For this review, take the finished solid that the model builds, in its own axes (mm). Coordinates: 2 decimals unless noted, no trailing zeros. Write each loop counter-clockwise with the first axis right and the second up, starting at its lowest first coordinate (ties: lowest second). Pieces come first, ordered by that corner, then holes. Notation, with made-up numbers: (-29, 33.5) -> (22, 33.5) arc R29 ccw to (22, 54.5) -> close; hole circle Ø1 at (-37, -15.5). An arc over 180 degrees is marked (long way). One line per item, written item: value. Start each with the question number.
1) Add section B-B (z = -226.5). State the section outline as (x, y) points, and give its area (3 significant figures).
2) For pin 1 Ø1.9 at (x, z) = (1.5, -552.5) entering from +Y; pin 2 Ø1.9 at (x, y) = (3, 617) entering from +Z, all flat-tipped, find the tip position at first contact; note any pin that passes through.
3) Add section A-A (x = 5). State how many separate pieces and enclosed holes the cut face has, and give its area (3 significant figures).
4) For probe 1 along Y at (x, z) = (1.75, -133.35); probe 2 along Y at (x, z) = (0.75, -596.5); probe 3 along Z at (x, y) = (5.75, 587), list the stretches that pass through material, from the lowest coordinate up. Write a range as from..to.
from build123d import *

# Parameters (mm, degrees)
SKETCH1_R           = 2.45745
BOSS_EXTRUDE1_DEPTH = 6.35
SKETCH3_R           = 2.45745
CUT_EXTRUDE2_DEPTH  = 1034.724611538


with BuildPart() as part:
    # Sketch1 → Boss-Extrude1 (new body)
    with BuildSketch(Plane(origin=(0, 0, 0), x_dir=(0, 0, -1), z_dir=(1, 0, 0))):
        with BuildLine():
            Line((457.2, 546.1), (755.65, 546.1))
            ThreePointArc((755.65, 546.1), (760.140128061, 544.240128061), (762, 539.75))
            Line((762, 539.75), (762, 6.35))
            ThreePointArc((762, 6.35), (760.140128061, 1.859871939), (755.65, 0))
            Line((755.65, 0), (6.35, 0))
            ThreePointArc((6.35, 0), (1.859871939, 1.859871939), (0, 6.35))
            Line((0, 6.35), (0, 539.75))
            ThreePointArc((0, 539.75), (1.859871939, 544.240128061), (6.35, 546.1))
            Line((6.35, 546.1), (304.8, 546.1))
            ThreePointArc((304.8, 546.1), (313.780256121, 549.819743879), (317.5, 558.8))
            Line((317.5, 558.8), (317.5, 685.8))
            ThreePointArc((317.5, 685.8), (321.219743879, 694.780256121), (330.2, 698.5))
            Line((330.2, 698.5), (431.8, 698.5))
            ThreePointArc((431.8, 698.5), (440.780256121, 694.780256121), (444.5, 685.8))
            Line((444.5, 685.8), (444.5, 558.8))
            ThreePointArc((444.5, 558.8), (448.219743879, 549.819743879), (457.2, 546.1))
        make_face()
        with Locations((53.975, 444.5)):
            Circle(SKETCH1_R, mode=Mode.SUBTRACT)
        with Locations((708.025, 444.5)):
            Circle(SKETCH1_R, mode=Mode.SUBTRACT)
        with Locations((708.025, 238.125)):
            Circle(SKETCH1_R, mode=Mode.SUBTRACT)
        with Locations((53.975, 238.125)):
            Circle(SKETCH1_R, mode=Mode.SUBTRACT)
        with Locations((53.975, 187.325)):
            Circle(SKETCH1_R, mode=Mode.SUBTRACT)
        with Locations((708.025, 187.325)):
            Circle(SKETCH1_R, mode=Mode.SUBTRACT)
    extrude(amount=BOSS_EXTRUDE1_DEPTH)

    # Sketch3 → Cut-Extrude2 (cut, through all)
    with BuildSketch(Plane(origin=(6.35, 0, 0), x_dir=(0, 0, -1), z_dir=(1, 0, 0))):
        with Locations((133.35, 415.925)):
            Circle(SKETCH3_R)
        with Locations((381, 415.925)):
            Circle(SKETCH3_R)
        with Locations((628.65, 415.925)):
            Circle(SKETCH3_R)
    extrude(amount=-CUT_EXTRUDE2_DEPTH, mode=Mode.SUBTRACT)


solid = part.part
Numbers:
1. outline: (0, 0) -> (6.35, 0) -> (6.35, 546.1) -> (0, 546.1) -> close
1. area: 3,470 mm²
2. pin 1: y = 546.1
2. pin 2: z = -317.5
3. separate pieces: 1
3. enclosed holes: 9
3. area: 435,000 mm²
4. probe 1: 0..413.47, 418.38..546.1
4. probe 2: 0..546.1
4. probe 3: -444.5..-317.5
